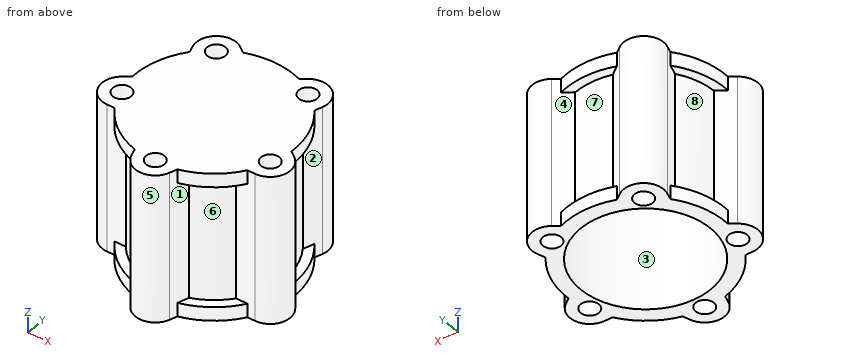
Autodesk Inventor part; units mm, degrees
ref_plane "YZ Plane" through (0, 0, 0) normal (1, 0, 0) x (0, 1, 0)
ref_plane "XZ Plane" through (0, 0, 0) normal (0, 1, 0) x (-1, 0, 0)
ref_plane "XY Plane" through (0, 0, 0) normal (0, 0, 1) x (1, 0, 0)
sketch "Sketch1" plane through (0, 0, 0) normal (0, 0, 1) x (1, 0, 0)
  circle A0 centre (0, 0) radius 77
  dimension "d0" = 154
extrude "Extrusion1" add sketch "Sketch1" along normal blind 162.5
shell "Shell1" thickness 6 removed faces 1 at (-19.0407, -8.1278, 0)
sketch "Sketch2" plane through (0, 0, 162.5) normal (0, 0, 1) x (1, 0, 0)
  circle A0 centre (0, 0) radius 87
  circle A1 centre (0, 0) radius 77
  dimension "d4" = 174
  dimension "d5" = 154
extrude "Extrusion2" add sketch "Sketch2" against normal blind 15
sketch "Sketch3" plane through (0, 0, 0) normal (0, 0, -1) x (-1, 0, 0)
  circle A0 centre (0, 0) radius 77
  circle A1 centre (0, 0) radius 87
extrude "Extrusion3" add sketch "Sketch3" against normal blind 15
sketch "Sketch4" plane through (0, 0, 0) normal (0, 0, -1) x (-1, 0, 0)
  arc A0 (70.6417, 62.0029) -> (37.1388, 86.3442) centre (49.9617, 68.7664) ccw
  line L0 (45.2595, 62.2943) -> (49.9617, 68.7664) construction
  line L1 (0, 77) -> (0, 87) construction
  line L2 (70.6417, 62.0029) -> (64.2451, 42.4448)
  arc A1 (68.0794, 54.1683) -> (30.4794, 81.4862) centre (0, 0) ccw construction
  arc A2 (68.0794, 54.1683) -> (30.4794, 81.4862) centre (0, 0) ccw construction
  circle A3 centre (0, 0) radius 77 construction
  circle A4 centre (0, 0) radius 77 construction
  arc A5 (64.2451, 42.4448) -> (-30.3958, 70.7467) centre (0, 0) ccw construction
  arc A6 (64.2451, 42.4448) -> (20.5146, 74.2169) centre (0, 0) ccw
  line L3 (20.5146, 74.2169) -> (37.1388, 86.3442)
  line L4 (76.9238, 3.4237) -> (93.5948, -8.6392)
  arc A7 (80.7978, -48.0243) -> (93.5948, -8.6392) centre (80.8398, -26.2664) ccw
  line L5 (80.7978, -48.0243) -> (60.2203, -47.9846)
  arc A8 (60.2203, -47.9846) -> (57.8913, 50.77) centre (0, 0) ccw construction
  line L6 (27.0269, -72.1009) -> (20.706, -91.6836)
  arc A9 (-20.706, -91.6836) -> (20.706, -91.6836) centre (0, -85) ccw
  line L7 (-20.706, -91.6836) -> (-27.0269, -72.1009)
  arc A10 (-27.0269, -72.1009) -> (66.1746, -39.3691) centre (0, 0) ccw construction
  line L8 (-60.2203, -47.9846) -> (-80.7978, -48.0243)
  arc A11 (-93.5948, -8.6392) -> (-80.7978, -48.0243) centre (-80.8398, -26.2664) ccw
  line L9 (-93.5948, -8.6392) -> (-76.9238, 3.4237)
  arc A12 (-76.9238, 3.4237) -> (-16.9932, -75.1015) centre (0, 0) ccw construction
  line L10 (-64.2451, 42.4448) -> (-70.6417, 62.0029)
  arc A13 (-37.1388, 86.3442) -> (-70.6417, 62.0029) centre (-49.9617, 68.7664) ccw
  line L11 (-37.1388, 86.3442) -> (-20.5146, 74.2169)
  arc A14 (-20.5146, 74.2169) -> (-76.6769, -7.0462) centre (0, 0) ccw construction
  point P0 (72.5548, -48.0084)
  point P1 (-23.2381, -83.8391)
  point P2 (-86.9167, -3.807)
  point P3 (-30.4794, 81.4862)
  dimension "d11" = 85
  dimension "d12" = 36
  dimension "d17" = 360
extrude "Extrusion4" add sketch "Sketch4" against normal blind 162.5
pattern_circular "Circular Pattern1" count 5 over 360 about axis through (0, 0, 0) along (0, 0, 1) of "Extrusion4"
sketch "Sketch5" plane through (0, 0, 0) normal (0, 0, -1) x (-1, 0, 0)
  arc A0 (70.6417, 62.0029) -> (37.1388, 86.3442) centre (49.9617, 68.7664) ccw construction
  circle A1 centre (49.9617, 68.7664) radius 10
  point P0 (0, 0)
  dimension "d22" = 20
extrude "Extrusion5" cut sketch "Sketch5" against normal up to next
pattern_circular "Circular Pattern2" count 5 over 360 about axis through (0, 0, 0) along (0, 0, 1) of "Extrusion5"
properties part number "inner"
Can you work these out from the model? Positions are in its coordinate system, mm. Face numbers are marked on the shaded views. A direction names the side the tool comes from. Round coordinates to 2 decimals unless told otherwise and drop trailing zeros. Loops run counter-clockwise (first coordinate to the right, second up) from the corner with the lowest first, then second, coordinate; pieces in that order, holes last. Notation, with made-up numbers: (74, 13) -> (82, 13) arc R14 ccw to (82, 23) -> close; hole circle Ø10 at (50, 50). An arc over 180 degrees is marked (long way). One line per item, written item: value. Start each with the question number.
1. If I drill on probe 1 along X at (y, z) = (72.5, 67); probe 2 along Y at (x, z) = (0.5, 60.5); probe 3 along Y at (x, z) = (-57.5, 109), over which ranges is the centre line in solid material (lowest first)?
2. If we mould it in two halves opening along X, with no side actions, what happens to the marked faces 6, 7 and 8? For each: pulls with the +X half, pulls with the -X half, needs draft (parallel to the pull), parting line crosses it, or undercut.
3. For pin 1 (4 mm diameter, centred on x = -34.5, z = 20.5, fed in from -Y); pin 2 (5 mm diameter, centred on x = 70.5, z = 97.5, fed in from -Y); pin 3 (8 mm diameter, centred on y = 55.5, z = 75.5, fed in from -X), each with a flat end and sliding along its axis, tell me the tip position at first contact or that it passes through.
4. If we section it at A-A, the plane y = -31.5: Write out the boundary of the cut face in (x, z), then the cut area to 3 significant figures.
5. For the marked faces 1, 2, 3, 4 and 5, which set-ups out of +Z, -Z, +X, -X, +Y, -Y let a thin tool reach every point of the face, with its end or its side?
6. If we section it at C-C, the plane y = -81: Write out the boundary of the cut face in (x, z).
7. If we section it at B-B, the plane x = 0: Write out the boundary of the cut face in (y, z), then the cut area to 3 significant figures.
Calculated:
1. probe 1: x = -71.4 to -59.24, -40.68 to 40.68, 59.24 to 71.4
1. probe 2: y = -106.75 to -94.99, -75.01 to -71, 71 to 77
1. probe 3: y = -51.21 to -41.65, 41.65 to 62.2, 75.34 to 89.18
2. face 6: pulls with the +X half
2. face 7: undercut
2. face 8: pulls with the -X half
3. pin 1: stops at y = -69.81
3. pin 2: stops at y = -48.01
3. pin 3: stops at x = -69.82
4. outline: (-101.96, 0) -> (-89.36, 0) -> (-89.36, 162.5) -> (-101.96, 162.5) -> close; (-72.32, 0) -> (-63.63, 0) -> (-63.63, 156.5) -> (63.63, 156.5) -> (63.63, 0) -> (72.32, 0) -> (72.32, 162.5) -> (-72.32, 162.5) -> close; (89.36, 0) -> (101.96, 0) -> (101.96, 162.5) -> (89.36, 162.5) -> close
4. area: 7,680 mm²
5. face 1: +X, -Y
5. face 2: +X
5. face 3: -Z
5. face 4: +Y
5. face 5: +Z, -Z, -Y
6. outline: (-31.75, 0) -> (-9.17, 0) -> (-9.17, 162.5) -> (-31.75, 162.5) -> (-31.75, 147.5) -> (-24.15, 147.5) -> (-24.15, 15) -> (-31.75, 15) -> close; (9.17, 0) -> (31.75, 0) -> (31.75, 15) -> (24.15, 15) -> (24.15, 147.5) -> (31.75, 147.5) -> (31.75, 162.5) -> (9.17, 162.5) -> close
7. outline: (-106.76, 0) -> (-95, 0) -> (-95, 162.5) -> (-106.76, 162.5) -> close; (-75, 0) -> (-71, 0) -> (-71, 156.5) -> (71, 156.5) -> (71, 0) -> (87, 0) -> (87, 15) -> (77, 15) -> (77, 147.5) -> (87, 147.5) -> (87, 162.5) -> (-75, 162.5) -> close
7. area: 4,690 mm²
